Here's how the part is built. I have some questions about the finished solid (model axes, mm). Give positions to 0.01 mm unless a question says otherwise; leave off trailing zeros. Order: outer loops, then holes, each group sorted by start corner. A loop starts at its lowest first (then second) coordinate and runs counter-clockwise, first axis right, second up. Notation, with made-up numbers: M 20.25,24 L 51.25,24 A30 ccw 51.25,58 Z; hole C 29.25,58 d4. An arc over 180 degrees is marked long. Use CSV: the item, a comma, the result in double quotes. Start each with the question number.
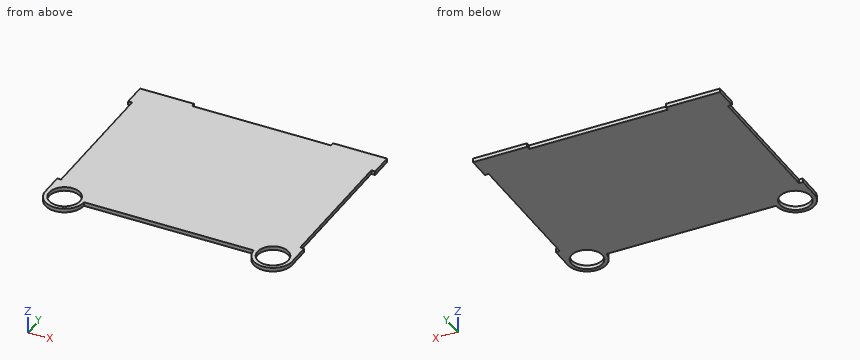
```python
from build123d import *

# Parameters (mm, degrees)
BOSS_EXTRUDE1_DEPTH     = 3.175
SKETCH2_R               = 12.7
CUT_EXTRUDE1_DEPTH      = 1
CUT_EXTRUDE1_DEPTH_BACK = 4.175
SKETCH3_W               = 3.175
SKETCH3_H               = 114.3
SKETCH3_W_2             = 114.3
SKETCH3_H_2             = 3.175
CUT_EXTRUDE2_DEPTH      = 4.175


with BuildPart() as part:
    # Sketch1 → Boss-Extrude1 (new body)
    with BuildSketch(Plane.XY):
        with BuildLine():
            Line((0, 0), (0, 152.4))
            Line((0, 152.4), (203.2, 152.4))
            Line((203.2, 152.4), (203.2, 0))
            ThreePointArc((203.2, 0), (187.325, -15.875), (171.45, 0))
            Line((171.45, 0), (31.75, 0))
            ThreePointArc((31.75, 0), (15.875, -15.875), (0, 0))
        make_face()
    extrude(amount=BOSS_EXTRUDE1_DEPTH)

    # Sketch2 → Cut-Extrude1 (cut, two sides)
    with BuildSketch(Plane.XY.offset(3.175)) as cut_extrude1_sk:
        with Locations((15.875, 0)):
            Circle(SKETCH2_R)
        with Locations((187.325, 0)):
            Circle(SKETCH2_R)
    extrude(amount=CUT_EXTRUDE1_DEPTH, mode=Mode.SUBTRACT)
    extrude(cut_extrude1_sk.sketch, amount=-CUT_EXTRUDE1_DEPTH_BACK, mode=Mode.SUBTRACT)

    # Sketch3 → Cut-Extrude2 (cut, through all)
    with BuildSketch(Plane.XY.offset(3.175)):
        with Locations((201.6125, 76.2)):
            Rectangle(SKETCH3_W, SKETCH3_H)
        with Locations((1.5875, 76.2)):
            Rectangle(SKETCH3_W, SKETCH3_H)
        with Locations((101.6, 150.8125)):
            Rectangle(SKETCH3_W_2, SKETCH3_H_2)
    extrude(amount=-CUT_EXTRUDE2_DEPTH, mode=Mode.SUBTRACT)


solid = part.part
```
Q1. I need wall thicknesses on line 1 (Y direction, x = 39, z = 2.85); line 2 (X direction, y = 127, z = 2.05) (3 decimals); line 3 (Y direction, x = 136, z = 2.3) (3 decimals). Which ranges of each line are inside material? Lowest first, please. Write a range as [from, to].
Q2. Imagine slicing it at C-C, the plane x = 136. Please give me the cut outline in (y, z) (3 decimals).
Q3. Imagine slicing it at D-D, the plane y = 33.5. Please give me the cut outline in (x, z) (3 decimals).
Q4. Imagine slicing it at B-B, the plane y = 4.5. Please give me the cut outline in (x, z) (3 decimals), then the cut area to 3 significant figures.
Q5. For P1, Ø1, axis at y = 63, z = 2.5, coming from the +X side (3 decimals); P2, Ø1.6, axis at x = 1, z = 1.5, coming from the -Y side; P3, Ø6, axis at x = 107, y = 134, coming from the -Z side, each with a flat end and sliding along its axis, tell me the tip position at first contact or that it passes through.
Q6. Imagine slicing it at A-A, the plane z = 1.75. Please give me the cut outline in (x, y) (3 decimals), then the cut area to 3 significant figures.
Reply:
1,line 1,"y = [0, 152.4]"
1,line 2,"x = [3.175, 200.025]"
1,line 3,"y = [0, 149.225]"
2,outline,"M 0,0 L 149.225,0 L 149.225,3.175 L 0,3.175 Z"
3,outline,"M 3.175,0 L 200.025,0 L 200.025,3.175 L 3.175,3.175 Z"
4,outline,"M 0,0 L 3.999,0 L 3.999,3.175 L 0,3.175 Z; M 27.751,0 L 175.449,0 L 175.449,3.175 L 27.751,3.175 Z; M 199.201,0 L 203.2,0 L 203.2,3.175 L 199.201,3.175 Z"
4,area,"494 mm^2"
5,P1,"stops at x = 200.025"
5,P2,"stops at y = -7.34"
5,P3,"stops at z = 0"
6,outline,"M 0,0 A15.875 ccw 31.75,0 L 171.45,0 A15.875 ccw 203.2,0 L 203.2,19.05 L 200.025,19.05 L 200.025,133.35 L 203.2,133.35 L 203.2,152.4 L 158.75,152.4 L 158.75,149.225 L 44.45,149.225 L 44.45,152.4 L 0,152.4 L 0,133.35 L 3.175,133.35 L 3.175,19.05 L 0,19.05 Z; hole C 15.875,0 d25.4; hole C 187.325,0 d25.4"
6,area,"29,700 mm^2"
